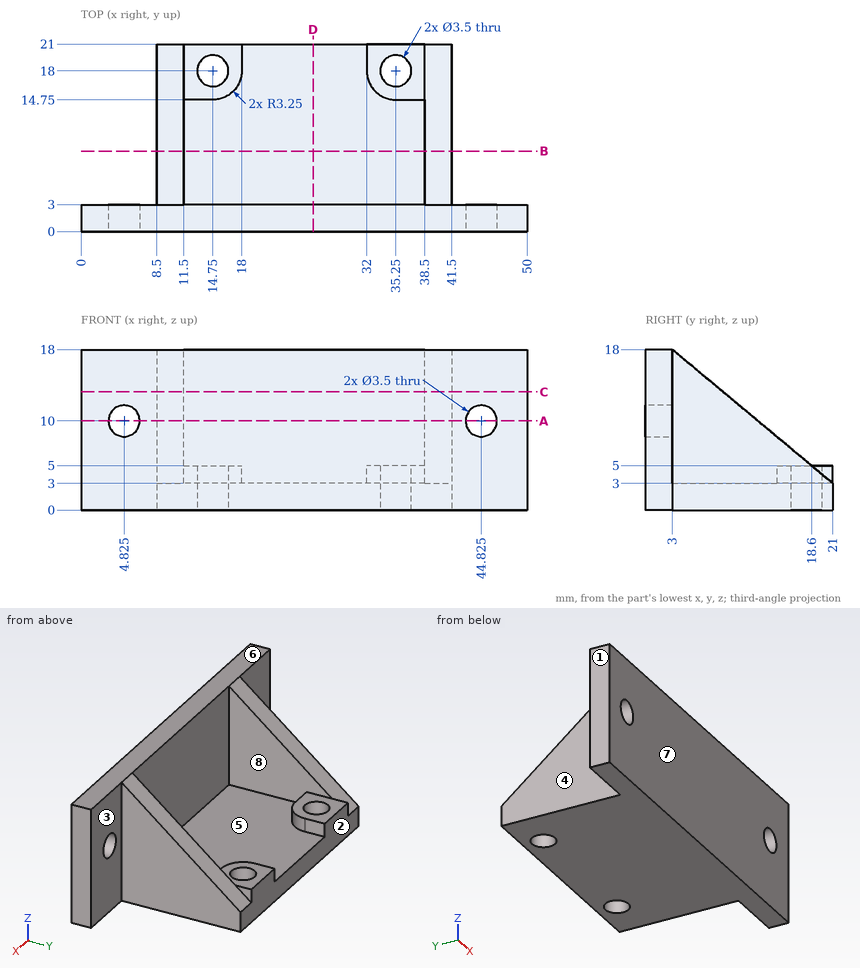
Study the drawing (mm; zero at the part's minimum x, y, z) and answer. A direction names the side the tool comes from. Round coordinates to 2 decimals unless told otherwise and drop trailing zeros. Write each loop counter-clockwise with the first axis right and the second up, starting at its lowest first coordinate (ties: lowest second). Pieces come first, ordered by that corner, then holes.
1) A tool of negligible diameter and unlimited length cuts with its end or side. For the marked faces 1, 2, 3, 4 and 5, from which of +Z, -Z, +X, -X, +Y, -Y can it reach the whole face along a straight path? Write none if from no direction.
2) Straight lines are drawn through the part: line 1 (X direction, y = 0.7, z = 10) (3 decimals); line 2 (Y direction, x = 35.25, z = 3.2); line 3 (X direction, y = 15.5, z = 6). For each, find the intervals that lie inside material, in ascending order.
3) The mould has two halves that part along Y. Classify the marked faces 6, 7 and 8: pulls with the +Y half, pulls with the -Y half, needs draft (parallel to the pull), parting line crosses it, or undercut.
4) A cutting plane is placed at B-B (y = 9). Give the vertices of the cut face in (x, z), plus the area to 3 significant figures.
5) Given pin 1 Ø7.5 at (x, z) = (29, 8.5) entering from +Y; pin 2 Ø8 at (y, z) = (15, 9) entering from +X; pin 3 Ø9 at (x, y) = (27, 10) entering from +Z, each flat-ended and moving along its own axis, determine where each tip first touches the part or whether it passes through.
6) A cutting plane is placed at A-A (z = 10). Give the vertices of the cut face in (x, y) (3 decimals).
7) A cutting plane is placed at C-C (z = 13.25). Give the vertices of the cut face in (x, y), plus the area to 3 significant figures.
8) A cutting plane is placed at D-D (x = 26). Give the vertices of the cut face in (y, z), plus the area to 3 significant figures.
Completed:
1. face 1: +Z, -Z, -X, +Y, -Y
1. face 2: +Z, -Z, +X, -X, +Y
1. face 3: +Z, -Z, +X, +Y
1. face 4: +Z, -Z, -X, +Y
1. face 5: +Z
2. line 1: x = 0 to 3.075, 6.575 to 43.075, 46.575 to 50
2. line 2: y = 0 to 3, 14.75 to 16.25, 19.75 to 21
2. line 3: x = 8.5 to 11.5, 38.5 to 41.5
3. face 6: needs draft
3. face 7: pulls with the -Y half
3. face 8: undercut
4. outline: (8.5, 0) - (41.5, 0) - (41.5, 13) - (38.5, 13) - (38.5, 3) - (11.5, 3) - (11.5, 13) - (8.5, 13) - close
4. area: 159 mm2
5. pin 1: stops at y = 3
5. pin 2: stops at x = 41.5
5. pin 3: stops at z = 3
6. outline: (0, 0) - (3.075, 0) - (3.075, 3) - (0, 3) - close; (6.575, 0) - (43.075, 0) - (43.075, 3) - (41.5, 3) - (41.5, 12.6) - (38.5, 12.6) - (38.5, 3) - (11.5, 3) - (11.5, 12.6) - (8.5, 12.6) - (8.5, 3) - (6.575, 3) - close; (46.575, 0) - (50, 0) - (50, 3) - (46.575, 3) - close
7. outline: (0, 0) - (50, 0) - (50, 3) - (41.5, 3) - (41.5, 8.7) - (38.5, 8.7) - (38.5, 3) - (11.5, 3) - (11.5, 8.7) - (8.5, 8.7) - (8.5, 3) - (0, 3) - close
7. area: 184 mm2
8. outline: (0, 0) - (21, 0) - (21, 3) - (3, 3) - (3, 18) - (0, 18) - close
8. area: 108 mm2
